from build123d import *

# Parameters (mm, degrees)
SKETCH1_R           = 18.5
BOSS_EXTRUDE1_DEPTH = 24
SKETCH2_R           = 16.5
BOSS_EXTRUDE2_DEPTH = 41
SKETCH6_R           = 1.25
CUT_EXTRUDE1_DEPTH  = 3.5
SKETCH7_R           = 6
BOSS_EXTRUDE5_DEPTH = 6
SKETCH8_R           = 3
BOSS_EXTRUDE6_DEPTH = 15
CUT_EXTRUDE2_START  = -12
CUT_EXTRUDE2_DEPTH  = 12
SKETCH3_W           = 4
SKETCH3_H           = 15
BOSS_EXTRUDE4_DEPTH = 8.763


with BuildPart() as part:
    # Sketch1 → Boss-Extrude1 (new body)
    with BuildSketch(Plane(origin=(0, 0, 0), x_dir=(1, 0, 0), z_dir=(0, 1, 0))):
        with Locations(Location((0, 0, 0), (0, 0, 270))):
            Circle(SKETCH1_R)
    extrude(amount=BOSS_EXTRUDE1_DEPTH)

    # Sketch2 → Boss-Extrude2 (add)
    with BuildSketch(Plane.XZ):
        with Locations(Location((0, 0, 0), (0, 0, 270))):
            Circle(SKETCH2_R)
    extrude(amount=BOSS_EXTRUDE2_DEPTH)

    # Sketch6 → Cut-Extrude1 (cut)
    with BuildSketch(Plane(origin=(0, 24, 0), x_dir=(1, 0, 0), z_dir=(0, 1, 0))):
        with Locations(Location((13.423393759, 7.75, 0), (0, 0, 270))):
            Circle(SKETCH6_R)
        with Locations(Location((0, 15.5, 0), (0, 0, 270))):
            Circle(SKETCH6_R)
        with Locations(Location((13.423393759, -7.75, 0), (0, 0, 270))):
            Circle(SKETCH6_R)
        with Locations(Location((0, -15.5, 0), (0, 0, 270))):
            Circle(SKETCH6_R)
        with Locations(Location((-13.423393759, -7.75, 0), (0, 0, 270))):
            Circle(SKETCH6_R)
        with Locations(Location((-13.423393759, 7.75, 0), (0, 0, 270))):
            Circle(SKETCH6_R)
    extrude(amount=-CUT_EXTRUDE1_DEPTH, mode=Mode.SUBTRACT)

    # Sketch7 → Boss-Extrude5 (add)
    with BuildSketch(Plane(origin=(0, 24, 0), x_dir=(1, 0, 0), z_dir=(0, 1, 0))):
        with Locations(Location((7, 0, 0), (0, 0, 270))):
            Circle(SKETCH7_R)
    extrude(amount=BOSS_EXTRUDE5_DEPTH)

    # Sketch8 → Boss-Extrude6 (add)
    with BuildSketch(Plane(origin=(0, 30, 0), x_dir=(1, 0, 0), z_dir=(0, 1, 0))):
        with Locations(Location((7, 0, 0), (0, 0, 270))):
            Circle(SKETCH8_R)
    extrude(amount=BOSS_EXTRUDE6_DEPTH)

    # Sketch9 → Cut-Extrude2 (cut)
    with BuildSketch(Plane(origin=(0, 45, 0), x_dir=(1, 0, 0), z_dir=(0, 1, 0)).offset(CUT_EXTRUDE2_START)):
        with BuildLine():
            Line((9.5, 1.658312395), (9.5, -1.658312395))
            ThreePointArc((9.5, -1.658312395), (10, 0), (9.5, 1.658312395))
        make_face()
    extrude(amount=CUT_EXTRUDE2_DEPTH, mode=Mode.SUBTRACT)

    # Sketch3 → Boss-Extrude4 (add, symmetric)
    with BuildSketch(Plane(origin=(16.249327925, 0, -2.865194932), x_dir=(0, 1, 0), z_dir=(0.984807753012208, 0, -0.17364817766693072))):
        with Locations((-30, 0.254363191)):
            Rectangle(SKETCH3_W, SKETCH3_H)
    extrude(amount=BOSS_EXTRUDE4_DEPTH, both=True)


solid = part.part
Work out the finished part from the listing and answer in its coordinate system (mm). A direction names the side the tool comes from. Give positions to 0.01 mm unless a question says otherwise; leave off trailing zeros. Loops run counter-clockwise (first coordinate to the right, second up) from the corner with the lowest first, then second, coordinate; pieces in that order, holes last. Notation, with made-up numbers: (14.25, -25.5) - (54.25, -25.5) arc R34 cw to (54.25, 8.5) - close; hole circle Ø5 at (32, 48.5). An arc over 180 degrees is marked (long way). Answer in a Markdown table with one row per item. Add a question column.
Q1. A tool of negligible diameter and unlimited length cuts with its end or side. For faces 4 (the flat face through (24.942, -30.028, -4.033)), 5 (the flat face through (21.031, -30.028, 4.166)), 6 (the flat face through (10, 30, 1)), 7 (the flat face through (9.5, 39, 0)), from which of +Z, -Z, +X, -X, +Y, -Y can it reach the whole face along a straight path? Write none if from no direction.
Q2. Determine the mould class of faces 1 (the cylindrical face through (4.07, 37.39, -0.65)), 2 (the cylindrical face through (-12.58, 22.27, 6.83)), 3 (the flat face through (0, 0, -17)) for opening direction X: released by +X, released by -X, zero draft, split by the parting line, or undercut.
Q3. The part is cut by section D-D (x = -6.5). Determine the outline of the cut face in (y, z).
Q4. The part is cut by section B-B (z = -7.75). Determine the outline of the cut face in (x, y), and give its area (3 significant figures).
Q5. The part is cut by section A-A (x = 0). Determine the outline of the cut face in (y, z).
Q6. Each of these flat-tipped pins is pushed along its axis until it touches: P1, Ø1.5, axis at x = 0, z = 15.5, coming from the +Y side; P2, Ø3, axis at x = 2.5, z = -9, coming from the +Y side; P3, Ø6, axis at x = 19, z = -8.5, coming from the -Y side. Where does it stop, or does it pass through?
Q7. Consider line 1 along Y through (x, z) = (-10, 8); line 2 along X through (y, z) = (23, -7); line 3 along X through (y, z) = (26.5, 0). Determine where each line is inside the solid, lowest interval first.
Q8. The part is cut by section C-C (y = 14.5). Determine the outline of the cut face in (x, z), and give its area (3 significant figures).
Solution:
| question | item | result |
|---|---|---|
| 1 | face 4 | -Z, +X, +Y, -Y |
| 1 | face 5 | +Z, +X, -Y |
| 1 | face 6 | +Y |
| 1 | face 7 | +Z, -Z, +X, +Y |
| 2 | face 1 | split by the parting line |
| 2 | face 2 | undercut |
| 2 | face 3 | zero draft |
| 3 | outline | (-41, -15.17) - (0, -15.17) - (0, -17.32) - (24, -17.32) - (24, 17.32) - (0, 17.32) - (0, 15.17) - (-41, 15.17) - close |
| 4 | outline | (-16.8, 0) - (-14.57, 0) - (-14.57, -41) - (14.57, -41) - (14.57, -32) - (24.29, -32) - (24.29, -28) - (14.57, -28) - (14.57, 0) - (16.8, 0) - (16.8, 24) - (14.67, 24) - (14.67, 20.5) - (12.17, 20.5) - (12.17, 24) - (-12.17, 24) - (-12.17, 20.5) - (-14.67, 20.5) - (-14.67, 24) - (-16.8, 24) - close |
| 4 | area | 2,020 mm² |
| 5 | outline | (-41, -16.5) - (0, -16.5) - (0, -18.5) - (24, -18.5) - (24, -16.75) - (20.5, -16.75) - (20.5, -14.25) - (24, -14.25) - (24, 14.25) - (20.5, 14.25) - (20.5, 16.75) - (24, 16.75) - (24, 18.5) - (0, 18.5) - (0, 16.5) - (-41, 16.5) - close |
| 6 | P1 | stops at y = 20.5 |
| 6 | P2 | stops at y = 24 |
| 6 | P3 | stops at y = -32 |
| 7 | line 1 | y = -41 to 24 |
| 7 | line 2 | x = -17.12 to -14.42, -12.42 to 12.42, 14.42 to 17.12 |
| 7 | line 3 | x = 1 to 13 |
| 8 | outline | circle Ø37 at (0, 0) |
| 8 | area | 1,080 mm² |
